Check sheet for the modelled part. Datum: model origin and axes. Units: mm. A direction names the side the tool comes from. Round coordinates to 2 decimals unless told otherwise and drop trailing zeros. Write each loop counter-clockwise with the first axis right and the second up, starting at its lowest first coordinate (ties: lowest second). Pieces come first, ordered by that corner, then holes. Notation, with made-up numbers: M 71,-31.75 L 129,-31.75 A34 ccw 129,5.25 Z; hole C 53.5,-39 d6. An arc over 180 degrees is marked long. Put each result on its own line as item: value.
```python
from build123d import *

# Parameters (mm, degrees)
F0_W     = 100
F0_H     = 100
F1_DEPTH = 100
F2_R     = 25
F3_DEPTH = 100
F5_DEPTH = 50


with BuildPart() as f1:
    # F0 (on Top) → F1 (new body)
    with BuildSketch(Plane.XY):
        Rectangle(F0_W, F0_H)
    extrude(amount=F1_DEPTH)

    # F2 (on face) → F3 (join)
    with BuildSketch(Plane(origin=(0, 0, 0), x_dir=(1, 0, 0), z_dir=(0, 0, -1))):
        Circle(F2_R)
    extrude(amount=F3_DEPTH)

    # F4 (on face) → F5 (cut)
    with BuildSketch(Plane.XZ.offset(50)):
        Polygon((12.5, 80.17767), (-12.5, 80.17767), (-30.17767, 62.5), (-30.17767, 37.5), (-12.5, 19.82233), (12.5, 19.82233), (30.17767, 37.5), (30.17767, 62.5), align=None)
    extrude(amount=-F5_DEPTH, mode=Mode.SUBTRACT)


solid = f1.part
```
1. Cross-section at C-C (z = -18). Enter the section's corners in (x, y), then the cut area to 3 significant figures.
Computed values:
outline: C 0,0 d50
area: 1,960 mm2
2. Release check for a two-part mould opening along Z. For faces 1 (the flat face through (-21.22, -25.35, 71.46)), 2 (the flat face through (0, 0, -100)), 3 (the cylindrical face through (23.846, -7.509, -49.3)) record: +Z half, -Z half, draft (parallel to the pull), parting line (faces both ways), or undercut.
Computed values:
face 1: undercut
face 2: -Z half
face 3: draft
3. Depth check by flat-ended pin: pin 1 Ø5 at (x, z) = (22.5, -13) entering from +Y; pin 2 Ø3 at (y, z) = (-11, -55.5) entering from +X; pin 3 Ø8 at (x, z) = (-12, -66.5) entering from -Y. Enter the tip coordinate at first touch or a pass-through.
Computed values:
pin 1: stops at y = 15
pin 2: stops at x = 23.12
pin 3: stops at y = -23.69
4. Scan lines: probe 1 along X at (y, z) = (-39, 62); probe 2 along Z at (x, y) = (3, -28.5); probe 3 along Y at (x, z) = (4.5, 55.5). Record each from-to range of solid material in increasing order.
Computed values:
probe 1: x = -50 to -30.18, 30.18 to 50
probe 2: z = 0 to 19.82, 80.18 to 100
probe 3: y = 0 to 50
5. Cross-section at B-B (x = -43). Enter the section's corners in (y, z), then the cut area to 3 significant figures.
Computed values:
outline: M -50,0 L 50,0 L 50,100 L -50,100 Z
area: 10,000 mm2
6. Access from +Z, -Z, +X, -X, +Y, -Y to the whole of each face (thin tool, end or side, straight path). Record for faces 4 (the flat face through (-12, 23, 0)), 5 (the flat face through (-30.178, -25, 50)), 6 (the flat face through (50, -1, 49)).
Computed values:
face 4: -Z
face 5: -Y
face 6: +Z, -Z, +X, +Y, -Y
7. Cross-section at A-A (y = -31.5). Enter the section's corners in (x, z), then the cut area to 3 significant figures.
Computed values:
outline: M -50,0 L 50,0 L 50,100 L -50,100 Z; hole M -30.18,37.5 L -12.5,19.82 L 12.5,19.82 L 30.18,37.5 L 30.18,62.5 L 12.5,80.18 L -12.5,80.18 L -30.18,62.5 Z
area: 6,980 mm2
